Geometry check sheet. Reference: drawing and pictorial views, mm from the part's lowest x, y, z. A direction names the side the tool comes from. Round coordinates to 2 decimals unless told otherwise and drop trailing zeros. Loops run counter-clockwise (first coordinate to the right, second up) from the corner with the lowest first, then second, coordinate; pieces in that order, holes last. Notation, with made-up numbers: (86.5, -27.5) - (127.5, -27.5) arc R35 ccw to (127.5, 11.5) - close; hole circle Ø4 at (-27.75, 60). An arc over 180 degrees is marked (long way). Answer as CSV lines item,"result". Start each with the question number.
1) Thickness scan on line 1 along X through (y, z) = (3.4, 4); line 2 along X through (y, z) = (2, 4); line 3 along Z through (x, y) = (90, 2.2). Record the ranges inside material, lowest first.
2) Cross-section at A-A on x = 52. Record the boundary of the cut face in (y, z), and give its area (3 significant figures).
3) Cross-section at B-B on y = 2.2. State how many separate pieces and enclosed holes the cut face has, and give its area (3 significant figures).
4) Cross-section at C-C on z = 7. Record the boundary of the cut face in (x, y), and give its area (3 significant figures).
5) Depth check by flat-ended pin: P1, Ø1.5, axis at x = 51.5, z = 4, coming from the +Y side; P2, Ø1, axis at y = 4.5, z = 5.5, coming from the +X side; P3, Ø1.8, axis at x = 3, z = 4, coming from the +Y side. Enter the tip coordinate at first touch or a pass-through.
6) Access from +Z, -Z, +X, -X, +Y, -Y to the whole of each face (thin tool, end or side, straight path). Record for the marked faces 1, 2 and 3.
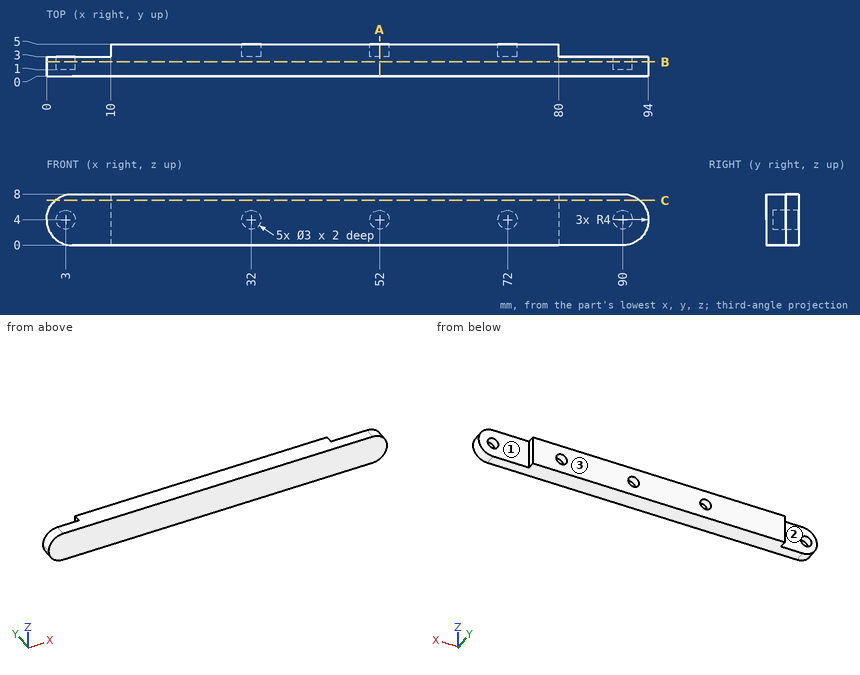
Answer block:
1,line 1,"x = 10 to 30.5, 33.5 to 50.5, 53.5 to 70.5, 73.5 to 80"
1,line 2,"x = 0 to 1.5, 4.5 to 88.5, 91.5 to 94"
1,line 3,"z = 0 to 2.5, 5.5 to 8"
2,outline,"(0, 0) - (5, 0) - (5, 2.5) - (3, 2.5) - (3, 5.5) - (5, 5.5) - (5, 8) - (0, 8) - close"
2,area,"34.0 mm^2"
3,separate pieces,"1"
3,enclosed holes,"2"
3,area,"724 mm^2"
4,outline,"(1.35, 0) - (92.65, 0) - (92.65, 3) - (80, 3) - (80, 5) - (10, 5) - (10, 3) - (1.35, 3) - close"
4,area,"414 mm^2"
5,P1,"stops at y = 3"
5,P2,"stops at x = 80"
5,P3,"stops at y = 1"
6,face 1,"+Z, -Z, +X, +Y"
6,face 2,"+Z, -Z, -X, +Y"
6,face 3,"+Z, -Z, +X, -X, +Y"
